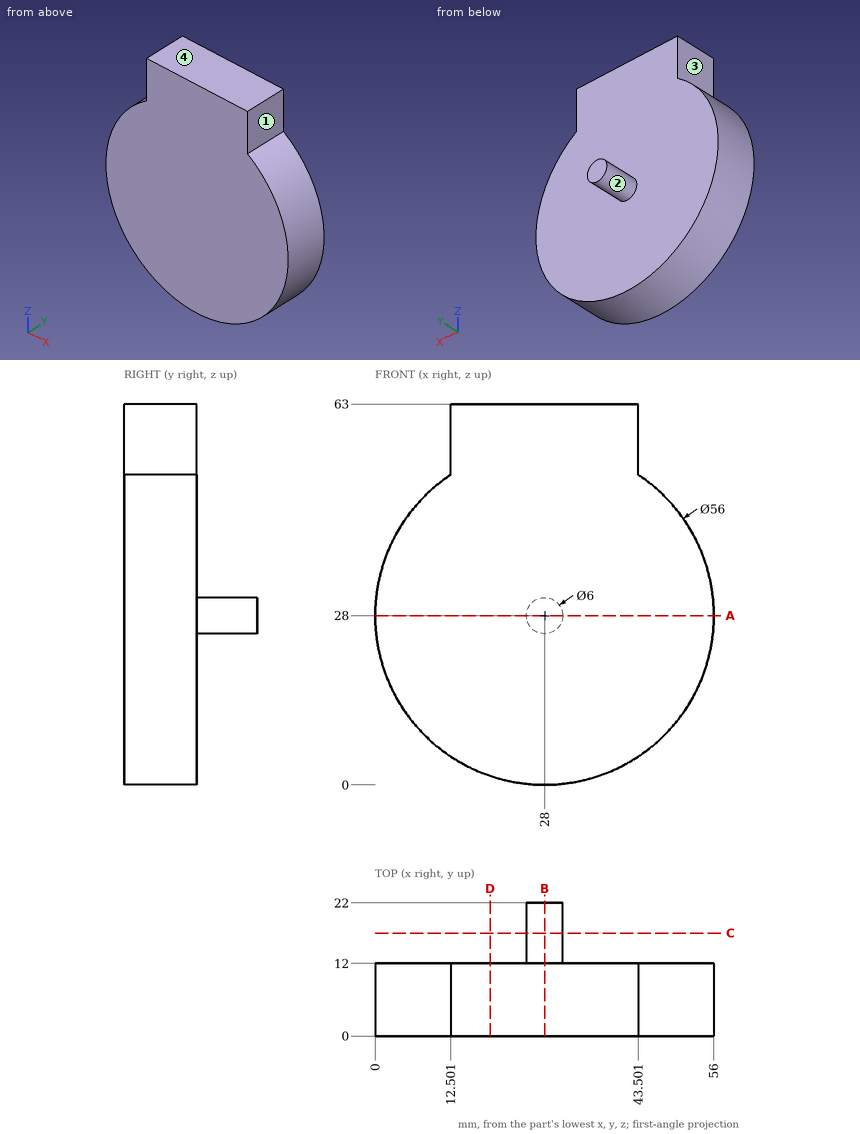
Input: dimensioned drawing with shaded views. Units: mm. Origin: part minimum x, y, z. A direction names the side the tool comes from. Give positions to 0.01 mm unless a question says otherwise; leave off trailing zeros. Write each loop counter-clockwise with the first axis right and the second up, starting at its lowest first coordinate (ties: lowest second). Pieces come first, ordered by that corner, then holes.
Q1. Set-up query: the marked faces 1, 2, 3 and 4. Return all of +Z, -Z, +X, -X, +Y, -Y with unobstructed straight access to the full face (end or side cutting, diameter ignored); none if empty.
Q2. Section C-C, the plane y = 17. Output: boundary loops of the cut face in (x, z).
Q3. Section D-D, the plane x = 19. Output: boundary loops of the cut face in (y, z), plus the area to 3 significant figures.
Q4. Section A-A, the plane z = 28. Output: boundary loops of the cut face in (x, y).
Q5. Section B-B, the plane x = 28. Output: boundary loops of the cut face in (y, z), plus the area to 3 significant figures.
Q6. Material intervals for probe 1 along Y at (x, z) = (15, 22); probe 2 along X at (y, z) = (7.5, 47.5); probe 3 along Z at (x, y) = (25.5, 17.5), sorted ascending.
Q7. First-contact query: P1, Ø10, axis at x = 7, z = 29.5, coming from the +Y side; P2, Ø4, axis at y = 10, z = 50.5, coming from the -X side; P3, Ø1.5, axis at x = 29, y = 8, coming from the -Z side. Flat tips, straight axial feed; report the tip coordinate or a pass-through.
Filled in:
1. face 1: +Z, +X, +Y, -Y
1. face 2: +Y
1. face 3: +Z, -X, +Y, -Y
1. face 4: +Z, +X, -X, +Y, -Y
2. outline: circle Ø6 at (28, 28)
3. outline: (0, 1.49) - (12, 1.49) - (12, 63) - (0, 63) - close
3. area: 738 mm2
4. outline: (0, 0) - (56, 0) - (56, 12) - (31, 12) - (31, 22) - (25, 22) - (25, 12) - (0, 12) - close
5. outline: (0, 0) - (12, 0) - (12, 25) - (22, 25) - (22, 31) - (12, 31) - (12, 63) - (0, 63) - close
5. area: 816 mm2
6. probe 1: y = 0 to 12
6. probe 2: x = 7.91 to 48.09
6. probe 3: z = 26.34 to 29.66
7. P1: stops at y = 12
7. P2: stops at x = 8.93
7. P3: stops at z = 0
